```python
from build123d import *

# Parameters (mm, degrees)
F0_W     = 193.9907595515
F0_H     = 168.106880039
F0_R     = 36.6772862691
F1_DEPTH = 127
F3_DEPTH = 25.4
F5_DEPTH = 168.106880039


with BuildPart() as f1:
    # F0 (on Right) → F1 (new body)
    with BuildSketch(Plane.YZ):
        with Locations((-10.7772685587, 24.0554083139)):
            Rectangle(F0_W, F0_H)
        with Locations((0, 18.1110166013)):
            Circle(F0_R, mode=Mode.SUBTRACT)
    extrude(amount=F1_DEPTH)

    # F2 (on face) → F3 (cut)
    with BuildSketch(Plane.XY.offset(108.1088483334)):
        with BuildLine():
            Line((0, 86.218111217), (0, 55.2217625082))
            add(Edge.make_bspline(
                [(0, 55.2217625082), (9.6147210988, 53.4978525461), (27.0066613183, 50.3794949053), (37.4402038298, 73.9035979944), (78.6246433045, 43.3299400269), (106.8380515, 63.040830288), (120.6463905868, 53.6422520116), (127, 49.3176989257)],
                knots=[0, 0, 0, 0, 0.1967507704, 0.3558998333, 0.6065111476, 0.8189445913, 1, 1, 1, 1], degree=3))
            Line((127, 49.3176989257), (127, 86.218111217))
            Line((127, 86.218111217), (0, 86.218111217))
        make_face()
    extrude(amount=-F3_DEPTH, mode=Mode.SUBTRACT)

    # F4 (on face) → F5 (cut, through all)
    with BuildSketch(Plane.XY.offset(108.1088483334)):
        Polygon((86.2131866927, -107.7726483345), (0, -14.5187666979), (0, -107.7726483345), align=None)
    extrude(amount=-F5_DEPTH, mode=Mode.SUBTRACT)


solid = f1.part
```
Could you check a few things on this model? Use its own coordinates, in mm. Coordinates: 2 decimals unless noted, no trailing zeros. Loops run counter-clockwise (first coordinate to the right, second up) from the corner with the lowest first, then second, coordinate; pieces in that order, holes last. Notation, with made-up numbers: M 89.5,87.25 L 147.5,87.25 A26 cw 147.5,105.25 Z; hole C -11.75,32.5 d6. An arc over 180 degrees is marked long. Put each result on its own line as item: value. Start each with the question number.
(1) Suppose I cut it at A-A on y = 0. Please give me the cut outline in (x, z), then the cut area to 3 significant figures.
(2) Suppose I cut it at B-B on z = 57.5. Please give me the cut outline in (x, y), then the cut area to 3 significant figures.
(3) Will this pin go through, and if not, where does the flat tip stop? P1, Ø12, axis at x = 21.5, z = -30, coming from the -Y side.
(4) I need wall thicknesses on line 1 (Z direction, x = 101, y = 0); line 2 (Y direction, x = 42.5, z = 23); line 3 (Y direction, x = 55, z = 2.5). Which ranges of each line are inside material? Lowest first, please. Write a range as from..to.
(5) Thinking about a two-plate mould opening in Z: for faces 1 (the face through (106, -107.773, 23)), 2 (the face through (63, 9, -59.998)), 3 (the face through (62.611, 34.984, 29.128)), which applies, pulls with the +Z half, pulls with the -Z half, needs draft (parallel to the pull), parting line crosses it, or undercut?
(6) Suppose I cut it at D-D on y = 68. Please give me the cut outline in (x, z), then the cut area to 3 significant figures.
(7) Suppose I cut it at C-C on z = 20.5. Please give me the cut outline in (x, y), then the cut area to 3 significant figures.
Solutions:
1. outline: M 0,-60 L 127,-60 L 127,-18.57 L 0,-18.57 Z; M 0,54.79 L 127,54.79 L 127,108.11 L 0,108.11 Z
1. area: 12,000 mm2
2. outline: M 0,-14.52 L 86.21,-107.77 L 127,-107.77 L 127,86.22 L 0,86.22 Z
2. area: 20,600 mm2
3. P1: stops at y = -44.26
4. line 1: z = -60..-18.57, 54.79..108.11
4. line 2: y = -60.49..-36.35, 36.35..86.22
4. line 3: y = -74.01..-33.19, 33.19..86.22
5. face 1: needs draft
5. face 2: pulls with the -Z half
5. face 3: undercut
6. outline: M 0,-60 L 127,-60 L 127,82.71 L 0,82.71 Z
6. area: 18,100 mm2
7. outline: M 0,36.6 L 127,36.6 L 127,86.22 L 0,86.22 Z; M 20.41,-36.6 L 86.21,-107.77 L 127,-107.77 L 127,-36.6 Z
7. area: 11,500 mm2
